Input: part model. Units: mm. Frame: model coordinates. Face numbers are marked on the shaded views. A direction names the side the tool comes from. Give positions to 0.01 mm unless a question says otherwise; leave off trailing zeros. Loops run counter-clockwise (first coordinate to the right, second up) from the corner with the lowest first, then second, coordinate; pieces in that order, holes last. Notation, with made-up numbers: M 64.5,56.25 L 73.5,56.25 A17 ccw 73.5,82.25 Z; hole C -4,-10.5 d8. An arc over 180 degrees is marked long. Use CSV: the item, a comma, the result in double quotes. Start each with the question number.
Q1. Section C-C, the plane x = 2.5. Output: boundary loops of the cut face in (y, z), plus the area to 3 significant figures.
Q2. Pull-direction query (Z, two-part tool) for the marked faces 3, 4 and 5; classes: released by +Z, released by -Z, zero draft, split by the parting line, or undercut.
Q3. Reachability of the marked faces 1 and 2 from +Z, -Z, +X, -X, +Y, -Y: full face, straight path, thin tool, end or side. Return the list, or none.
Q4. Material intervals for line 1 along Y through (x, z) = (12.75, -0.5); line 2 along X through (y, z) = (-11, -3.5); line 3 along Z through (x, y) = (7.75, -0.5), sorted ascending.
Q5. Pin query (flat end, axial travel): pin 1 (3 mm diameter, centred on x = 6, y = 0, fed in from +Z); pin 2 (5.5 mm diameter, centred on y = -6, z = -10.39, fed in from -X); pin 3 (3 mm diameter, centred on x = 2, y = 3, fed in from +Z). Return the tip coordinate at first contact, or that it passes through.
Q6. Section B-B, the plane y = 0. Output: boundary loops of the cut face in (x, z).
Q7. Section A-A, the plane z = 0. Output: boundary loops of the cut face in (x, y), plus the area to 3 significant figures.
Q8. Section D-D, the plane x = 12.75. Output: boundary loops of the cut face in (y, z).
from build123d import *

# Parameters (mm, degrees)
ESQUISSE2_R                  = 1.25
ENL_V_MAT_EXTRU_1_DEPTH      = 30.051678093
TROU_TARAUD_M41_D            = 3.3
R_P_TITION_CIRCULAIRE1_COUNT = 3
CHANFREIN1_SIZE              = 0.6


with BuildPart() as part:
    # Esquisse1 → Révolution1 (revolve)
    with BuildSketch(Plane.XY, mode=Mode.PRIVATE) as r_volution1_sk:
        Polygon((0, 3), (14, 3), (14, 18), (9, 18), (9, 7.5), (0, 7.5), align=None)
    revolve(r_volution1_sk.sketch.rotate(Axis((0, 0, 0), (1, 0, 0)), 90), axis=Axis((0, 0, 0), (1, 0, 0)))

    # Esquisse2 → Enlèv. mat.-Extru.1 (cut, through all)
    with BuildSketch(Plane.XY):
        with Locations((6, 0)):
            Circle(ESQUISSE2_R)
    extrude(amount=-ENL_V_MAT_EXTRU_1_DEPTH, mode=Mode.SUBTRACT)

    # Trou taraudé M41 (through all)
    with Locations(Plane(origin=(14, 0, 0), x_dir=(0, 0, -1), z_dir=(1, 0, 0))):
        with Locations((0, 12)):
            trou_taraud_m41 = Hole(TROU_TARAUD_M41_D / 2)

    # Répétition circulaire1: Trou taraudé M41 ×3 about axis
    r_p_tition_circulaire1_axis = Axis((0, 0, 0), (1, 0, 0))
    for i in range(1, R_P_TITION_CIRCULAIRE1_COUNT):
        add(trou_taraud_m41.rotate(r_p_tition_circulaire1_axis, i * 360 / R_P_TITION_CIRCULAIRE1_COUNT), mode=Mode.SUBTRACT)

    # Chanfrein1
    chanfrein1_edges = [part.edges().sort_by_distance(p)[0] for p in [
        (14, 0, -18),
    ]]
    chamfer(chanfrein1_edges, length=CHANFREIN1_SIZE)


solid = part.part
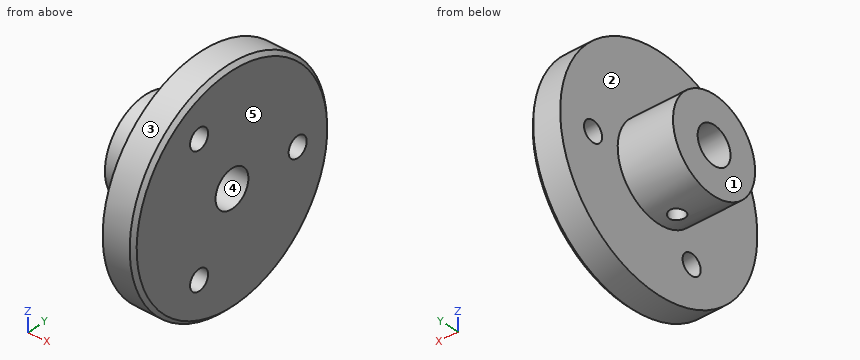
A:
1,outline,"C 0,0 d15; hole C 0,0 d6"
1,area,"148 mm^2"
2,face 3,"split by the parting line"
2,face 4,"undercut"
2,face 5,"zero draft"
3,face 1,"+Z, -Z, -X, +Y, -Y"
3,face 2,"-X"
4,line 1,"-17.99 to -2.96, 2.96 to 10.43, 13.57 to 17.99"
4,line 2,"9 to 14"
4,line 3,"-7.48 to -2.96, 2.96 to 7.48"
5,pin 1,"z = 7.5"
5,pin 2,"x = 9"
5,pin 3,"z = 7.35"
6,outline,"M 0,-7.5 L 4.75,-7.5 L 4.75,-3 L 0,-3 Z; M 0,3 L 14,3 L 14,17.4 L 13.4,18 L 9,18 L 9,7.5 L 0,7.5 Z; M 7.25,-7.5 L 9,-7.5 L 9,-18 L 13.4,-18 L 14,-17.4 L 14,-3 L 7.25,-3 Z"
7,outline,"M 0,-7.5 L 9,-7.5 L 9,-18 L 13.4,-18 L 14,-17.4 L 14,-3 L 0,-3 Z; M 0,3 L 14,3 L 14,10.35 L 9,10.35 L 9,7.5 L 0,7.5 Z; M 9,13.65 L 14,13.65 L 14,17.4 L 13.4,18 L 9,18 Z"
7,area,"214 mm^2"
8,outline,"C 0,0 d36; hole C -6,-10.39 d3.3; hole C -6,10.39 d3.3; hole C 0,0 d6; hole C 12,0 d3.3"
